Can you work these out from the model? Positions are in its coordinate system, mm. A direction names the side the tool comes from. Give positions to 0.01 mm unless a question says otherwise; leave off trailing zeros. Loops run counter-clockwise (first coordinate to the right, second up) from the corner with the lowest first, then second, coordinate; pieces in that order, holes last. Notation, with made-up numbers: (77, 57.5) - (131, 57.5) arc R23 cw to (131, 79.5) - close; hole circle Ø6 at (-9, 52). An arc over 180 degrees is marked (long way). Answer in a Markdown table with one row per item.
from build123d import *

# Parameters (mm, degrees)
SKETCH1_W            = 6.6
SKETCH1_H            = 11.95
BOSS_EXTRUDE1_DEPTH  = 5
SKETCH2_W            = 3.4
SKETCH2_H            = 0.5
CUT_EXTRUDE1_DEPTH   = 1.4
SKETCH3_W            = 2.2
SKETCH3_H            = 0.65
CUT_EXTRUDE2_DEPTH   = 7.1
SKETCH4_W            = 2.2
SKETCH4_H            = 0.25
BOSS_EXTRUDE2_DEPTH  = 0.5
SKETCH5_W            = 2.2
SKETCH5_H            = 0.25
BOSS_EXTRUDE3_DEPTH  = 0.6
SKETCH6_W            = 3.4
SKETCH6_H            = 0.5
CUT_EXTRUDE3_DEPTH   = 1.4
SKETCH7_W            = 2.2
SKETCH7_H            = 0.65
CUT_EXTRUDE4_DEPTH   = 7.1
SKETCH8_W            = 2.2
SKETCH8_H            = 0.25
BOSS_EXTRUDE4_DEPTH  = 0.5
SKETCH9_W            = 2.2
SKETCH9_H            = 0.25
BOSS_EXTRUDE5_DEPTH  = 0.6
CUT_EXTRUDE5_DEPTH   = 3.6
CUT_EXTRUDE6_REACH   = 2.9
SKETCH12_W           = 2.2
SKETCH12_H           = 2.6
CUT_EXTRUDE7_REACH   = 12.275
SKETCH13_W           = 1.85
SKETCH13_H           = 4.85
SKETCH14_W           = 2.5
SKETCH14_H           = 4.25
CUT_EXTRUDE8_DEPTH   = 1.65
CUT_EXTRUDE9_REACH   = 2.9
SKETCH16_W           = 2.2
SKETCH16_H           = 2.6
CUT_EXTRUDE10_REACH  = 12.275
SKETCH17_W           = 1.85
SKETCH17_H           = 4.85
SKETCH18_W           = 2.5
SKETCH18_H           = 4.25
CUT_EXTRUDE11_DEPTH  = 1.65
CUT_EXTRUDE12_REACH  = 6.85
SKETCH20_W           = 0.8
SKETCH20_H           = 3.6
SKETCH21_W           = 0.8
SKETCH21_H           = 1.9
CUT_EXTRUDE13_DEPTH  = 2.675
SKETCH22_W           = 0.8
SKETCH22_H           = 1.9
CUT_EXTRUDE14_DEPTH  = 2.675
SKETCH23_W           = 0.5
SKETCH23_H           = 0.5
BOSS_EXTRUDE6_DEPTH  = 2
SKETCH24_W           = 0.5
SKETCH24_H           = 0.5
BOSS_EXTRUDE7_DEPTH  = 2
SKETCH25_W           = 0.5
SKETCH25_H           = 0.5
BOSS_EXTRUDE8_DEPTH  = 2
SKETCH26_W           = 0.5
SKETCH26_H           = 0.5
BOSS_EXTRUDE9_DEPTH  = 2
SKETCH27_W           = 0.5
SKETCH27_H           = 0.5
BOSS_EXTRUDE10_DEPTH = 3.3
SKETCH28_W           = 0.5
SKETCH28_H           = 0.5
BOSS_EXTRUDE11_DEPTH = 3.3
SKETCH29_W           = 0.5
SKETCH29_H           = 0.5
BOSS_EXTRUDE12_DEPTH = 3.3
SKETCH30_W           = 0.5
SKETCH30_H           = 0.5
BOSS_EXTRUDE13_DEPTH = 3.3
DRAFT1_ANGLE         = 45


with BuildPart() as part:
    # Sketch1 → Boss-Extrude1 (new body)
    with BuildSketch(Plane(origin=(-5, 0, 0), x_dir=(0, -1, 0), z_dir=(-1, 0, 0))):
        with Locations((-3.3, 0)):
            Rectangle(SKETCH1_W, SKETCH1_H)
    extrude(amount=-BOSS_EXTRUDE1_DEPTH)

    # Sketch2 → Cut-Extrude1 (cut)
    with BuildSketch(Plane.XY.offset(5.975)):
        with Locations((-2.5, 0.25)):
            Rectangle(SKETCH2_W, SKETCH2_H)
    extrude(amount=-CUT_EXTRUDE1_DEPTH, mode=Mode.SUBTRACT)

    # Sketch3 → Cut-Extrude2 (cut, through all)
    with BuildSketch(Plane.XZ.offset(-0.5)):
        with Locations((-2.5, 5.65)):
            Rectangle(SKETCH3_W, SKETCH3_H)
    extrude(amount=-CUT_EXTRUDE2_DEPTH, mode=Mode.SUBTRACT)

    # Sketch4 → Boss-Extrude2 (add)
    with BuildSketch(Plane.XZ.offset(-0.5)):
        with Locations((-2.5, 5.2)):
            Rectangle(SKETCH4_W, SKETCH4_H)
    extrude(amount=BOSS_EXTRUDE2_DEPTH)

    # Sketch5 → Boss-Extrude3 (add)
    with BuildSketch(Plane.XY.offset(5.325)):
        with Locations((-2.5, 0.125)):
            Rectangle(SKETCH5_W, SKETCH5_H)
    extrude(amount=BOSS_EXTRUDE3_DEPTH)

    # Sketch6 → Cut-Extrude3 (cut)
    with BuildSketch(Plane(origin=(0, 0, -5.975), x_dir=(-1, 0, 0), z_dir=(0, 0, -1))):
        with Locations((2.5, 0.25)):
            Rectangle(SKETCH6_W, SKETCH6_H)
    extrude(amount=-CUT_EXTRUDE3_DEPTH, mode=Mode.SUBTRACT)

    # Sketch7 → Cut-Extrude4 (cut, through all)
    with BuildSketch(Plane.XZ.offset(-0.5)):
        with Locations((-2.5, -5.65)):
            Rectangle(SKETCH7_W, SKETCH7_H)
    extrude(amount=-CUT_EXTRUDE4_DEPTH, mode=Mode.SUBTRACT)

    # Sketch8 → Boss-Extrude4 (add)
    with BuildSketch(Plane.XZ.offset(-0.5)):
        with Locations((-2.5, -5.2)):
            Rectangle(SKETCH8_W, SKETCH8_H)
    extrude(amount=BOSS_EXTRUDE4_DEPTH)

    # Sketch9 → Boss-Extrude5 (add)
    with BuildSketch(Plane(origin=(0, 0, -5.325), x_dir=(-1, 0, 0), z_dir=(0, 0, -1))):
        with Locations((2.5, 0.125)):
            Rectangle(SKETCH9_W, SKETCH9_H)
    extrude(amount=BOSS_EXTRUDE5_DEPTH)

    # Sketch10 → Cut-Extrude5 (cut)
    with BuildSketch(Plane(origin=(0, 0, -1.8), x_dir=(-1, 0, 0), z_dir=(0, 0, -1))):
        Polygon((5, 2.35), (5, 6.6), (0.7, 6.6), (0.7, 1.75), (2.55, 1.75), (2.55, 2.35), align=None)
    extrude(amount=-CUT_EXTRUDE5_DEPTH, mode=Mode.SUBTRACT)

    # Sketch12 → Cut-Extrude6 (cut, up to next)
    with BuildSketch(Plane(origin=(0, 0, 5.075), x_dir=(-1, 0, 0), z_dir=(0, 0, -1)), mode=Mode.PRIVATE) as cut_extrude6_sk1:
        with Locations((2.5, 5.3)):
            Rectangle(SKETCH12_W, SKETCH12_H)
    cut_extrude6_tool1 = extrude(cut_extrude6_sk1.sketch, amount=-CUT_EXTRUDE6_REACH, mode=Mode.PRIVATE) & part.part
    add(cut_extrude6_tool1.solids().sort_by_distance((-2.5, 5.3, 5.075))[0], mode=Mode.SUBTRACT)

    # Sketch13 → Cut-Extrude7 (cut, up to next)
    with BuildSketch(Plane.XY.offset(4.3), mode=Mode.PRIVATE) as cut_extrude7_sk1:
        with Locations((-1.625, 4.175)):
            Rectangle(SKETCH13_W, SKETCH13_H)
    cut_extrude7_tool1 = extrude(cut_extrude7_sk1.sketch, amount=-CUT_EXTRUDE7_REACH, mode=Mode.PRIVATE) & part.part
    add(cut_extrude7_tool1.solids().sort_by_distance((-1.625, 4.175, 4.3))[0], mode=Mode.SUBTRACT)

    # Sketch14 → Cut-Extrude8 (cut)
    with BuildSketch(Plane(origin=(-2.55, 0, 0), x_dir=(0, 0, -1), z_dir=(1, 0, 0))):
        with Locations((-3.05, 4.475)):
            Rectangle(SKETCH14_W, SKETCH14_H)
    extrude(amount=-CUT_EXTRUDE8_DEPTH, mode=Mode.SUBTRACT)

    # Sketch16 → Cut-Extrude9 (cut, up to next)
    with BuildSketch(Plane.XY.offset(-5.075), mode=Mode.PRIVATE) as cut_extrude9_sk1:
        with Locations((-2.5, 5.3)):
            Rectangle(SKETCH16_W, SKETCH16_H)
    cut_extrude9_tool1 = extrude(cut_extrude9_sk1.sketch, amount=-CUT_EXTRUDE9_REACH, mode=Mode.PRIVATE) & part.part
    add(cut_extrude9_tool1.solids().sort_by_distance((-2.5, 5.3, -5.075))[0], mode=Mode.SUBTRACT)

    # Sketch17 → Cut-Extrude10 (cut, up to next)
    with BuildSketch(Plane(origin=(0, 0, -4.3), x_dir=(-1, 0, 0), z_dir=(0, 0, -1)), mode=Mode.PRIVATE) as cut_extrude10_sk1:
        with Locations((1.625, 4.175)):
            Rectangle(SKETCH17_W, SKETCH17_H)
    cut_extrude10_tool1 = extrude(cut_extrude10_sk1.sketch, amount=-CUT_EXTRUDE10_REACH, mode=Mode.PRIVATE) & part.part
    add(cut_extrude10_tool1.solids().sort_by_distance((-1.625, 4.175, -4.3))[0], mode=Mode.SUBTRACT)

    # Sketch18 → Cut-Extrude11 (cut)
    with BuildSketch(Plane(origin=(-2.55, 0, 0), x_dir=(0, 0, -1), z_dir=(1, 0, 0))):
        with Locations((3.05, 4.475)):
            Rectangle(SKETCH18_W, SKETCH18_H)
    extrude(amount=-CUT_EXTRUDE11_DEPTH, mode=Mode.SUBTRACT)

    # Sketch20 → Cut-Extrude12 (cut, up to next)
    with BuildSketch(Plane.XZ.offset(-1.75), mode=Mode.PRIVATE) as cut_extrude12_sk1:
        with Locations((-4.6, 0)):
            Rectangle(SKETCH20_W, SKETCH20_H)
    cut_extrude12_tool1 = extrude(cut_extrude12_sk1.sketch, amount=-CUT_EXTRUDE12_REACH, mode=Mode.PRIVATE) & part.part
    add(cut_extrude12_tool1.solids().sort_by_distance((-4.6, 1.75, 0))[0], mode=Mode.SUBTRACT)

    # Sketch21 → Cut-Extrude13 (cut, through all)
    with BuildSketch(Plane(origin=(0, 0, 4.3), x_dir=(-1, 0, 0), z_dir=(0, 0, -1))):
        with Locations((2.95, 5.65)):
            Rectangle(SKETCH21_W, SKETCH21_H)
    extrude(amount=-CUT_EXTRUDE13_DEPTH, mode=Mode.SUBTRACT)

    # Sketch22 → Cut-Extrude14 (cut, through all)
    with BuildSketch(Plane.XY.offset(-4.3)):
        with Locations((-2.95, 5.65)):
            Rectangle(SKETCH22_W, SKETCH22_H)
    extrude(amount=-CUT_EXTRUDE14_DEPTH, mode=Mode.SUBTRACT)

    # Sketch23 → Boss-Extrude6 (add)
    with BuildSketch(Plane(origin=(0, 0, 0), x_dir=(0, 0, -1), z_dir=(1, 0, 0))):
        with Locations((-3, 0.25)):
            Rectangle(SKETCH23_W, SKETCH23_H)
    extrude(amount=BOSS_EXTRUDE6_DEPTH)

    # Sketch24 → Boss-Extrude7 (add)
    with BuildSketch(Plane(origin=(0, 0, 0), x_dir=(0, 0, -1), z_dir=(1, 0, 0))):
        with Locations((-1, 0.25)):
            Rectangle(SKETCH24_W, SKETCH24_H)
    extrude(amount=BOSS_EXTRUDE7_DEPTH)

    # Sketch25 → Boss-Extrude8 (add)
    with BuildSketch(Plane(origin=(0, 0, 0), x_dir=(0, 0, -1), z_dir=(1, 0, 0))):
        with Locations((1, 0.25)):
            Rectangle(SKETCH25_W, SKETCH25_H)
    extrude(amount=BOSS_EXTRUDE8_DEPTH)

    # Sketch26 → Boss-Extrude9 (add)
    with BuildSketch(Plane(origin=(0, 0, 0), x_dir=(0, 0, -1), z_dir=(1, 0, 0))):
        with Locations((3, 0.25)):
            Rectangle(SKETCH26_W, SKETCH26_H)
    extrude(amount=BOSS_EXTRUDE9_DEPTH)

    # Sketch27 → Boss-Extrude10 (add)
    with BuildSketch(Plane(origin=(0, 2.35, 0), x_dir=(-1, 0, 0), z_dir=(0, 1, 0))):
        with Locations((3.1, -3)):
            Rectangle(SKETCH27_W, SKETCH27_H)
    extrude(amount=BOSS_EXTRUDE10_DEPTH)

    # Sketch28 → Boss-Extrude11 (add)
    with BuildSketch(Plane(origin=(0, 2.35, 0), x_dir=(-1, 0, 0), z_dir=(0, 1, 0))):
        with Locations((3.1, -1)):
            Rectangle(SKETCH28_W, SKETCH28_H)
    extrude(amount=BOSS_EXTRUDE11_DEPTH)

    # Sketch29 → Boss-Extrude12 (add)
    with BuildSketch(Plane(origin=(0, 2.35, 0), x_dir=(-1, 0, 0), z_dir=(0, 1, 0))):
        with Locations((3.1, 1)):
            Rectangle(SKETCH29_W, SKETCH29_H)
    extrude(amount=BOSS_EXTRUDE12_DEPTH)

    # Sketch30 → Boss-Extrude13 (add)
    with BuildSketch(Plane(origin=(0, 2.35, 0), x_dir=(-1, 0, 0), z_dir=(0, 1, 0))):
        with Locations((3.1, 3)):
            Rectangle(SKETCH30_W, SKETCH30_H)
    extrude(amount=BOSS_EXTRUDE13_DEPTH)

    # Draft1
    draft1_faces = [part.faces().sort_by_distance(p)[0] for p in [
        (-2.55, 2.05, 0),
    ]]
    draft(draft1_faces, Plane(origin=(-2.55, 2.35, 1.8), x_dir=(0, 0, 1), z_dir=(0, 1, 0)), DRAFT1_ANGLE)


solid = part.part
Q1. If I drill on line 1 (X direction, y = 5, z = -3); line 2 (X direction, y = 2.5, z = -2.25); line 3 (Z direction, x = -4.25, y = 2) (3 decimals), over which ranges is the centre line in solid material (lowest first)? Write a range as [from, to].
Checked values:
| item | result |
|---|---|
| line 1 | x = [-5, -4.2], [-3.35, -2.85], [-0.7, 0] |
| line 2 | x = [-5, -4.2], [-0.7, 0] |
| line 3 | z = [-5.975, -1.8], [1.8, 5.975] |
Q2. Imagine slicing it at D-D, the plane z = -0.25. Write out the boundary of the cut face in (x, y), and give its area (3 significant figures).
Checked values:
| item | result |
|---|---|
| outline | (-5, 0) - (0, 0) - (0, 6.6) - (-0.7, 6.6) - (-0.7, 1.75) - (-1.95, 1.75) - (-2.55, 2.35) - (-4.2, 2.35) - (-4.2, 1.75) - (-5, 1.75) - close |
| area | 13.3 mm² |
Q3. Imagine slicing it at B-B, the plane y = 6. Write out the boundary of the cut face in (x, z) (3 decimals).
Checked values:
| item | result |
|---|---|
| outline | (-5, -5.975) - (-3.6, -5.975) - (-3.6, -5.075) - (-3.35, -5.075) - (-3.35, -4.3) - (-4.2, -4.3) - (-4.2, -1.8) - (-5, -1.8) - close; (-5, 1.8) - (-4.2, 1.8) - (-4.2, 4.3) - (-3.35, 4.3) - (-3.35, 5.075) - (-3.6, 5.075) - (-3.6, 5.975) - (-5, 5.975) - close; (-2.55, -5.075) - (-1.4, -5.075) - (-1.4, -5.975) - (0, -5.975) - (0, 5.975) - (-1.4, 5.975) - (-1.4, 5.075) - (-2.55, 5.075) - (-2.55, 4.3) - (-0.7, 4.3) - (-0.7, -4.3) - (-2.55, -4.3) - close |
Q4. On a 3-axis mill with a long thin cutter (end or side, diameter ignored), from which of +Z, -Z, +X, -X, +Y, -Y can I reach the whole of each face in a straight line? I mean faces 1 (the face through (-0.7, 4, 0)), 2 (the face through (-1.4, 3.5, -5.5)), 3 (the face through (-4.6, 1.75, 0)). Say none if no direction works.
Checked values:
| item | result |
|---|---|
| face 1 | +Y |
| face 2 | -Z, +Y |
| face 3 | -X, +Y |
Q5. Imagine slicing it at A-A, the plane x = 1.25. Write out the boundary of the cut face in (y, z), and give its area (3 significant figures).
Checked values:
| item | result |
|---|---|
| outline | (0, -3.25) - (0.5, -3.25) - (0.5, -2.75) - (0, -2.75) - close; (0, -1.25) - (0.5, -1.25) - (0.5, -0.75) - (0, -0.75) - close; (0, 0.75) - (0.5, 0.75) - (0.5, 1.25) - (0, 1.25) - close; (0, 2.75) - (0.5, 2.75) - (0.5, 3.25) - (0, 3.25) - close |
| area | 1.00 mm² |
Q6. Imagine slicing it at C-C, the plane y = 1.5. Write out the boundary of the cut face in (x, z) (3 decimals).
Checked values:
| item | result |
|---|---|
| outline | (-5, -5.975) - (-3.6, -5.975) - (-3.6, -5.325) - (-1.4, -5.325) - (-1.4, -5.975) - (0, -5.975) - (0, 5.975) - (-1.4, 5.975) - (-1.4, 5.325) - (-3.6, 5.325) - (-3.6, 5.975) - (-5, 5.975) - close |
Q7. If we mould it in two halves opening along Z, with no side actions, what happens to faces 4 (the face through (-1, 3, -5.975)), 5 (the face through (-4.2, 5, 3)), 6 (the face through (-4.4, 6.6, -4.4))? For each: released by +Z, released by -Z, zero draft, split by the parting line, or undercut.
Checked values:
| item | result |
|---|---|
| face 4 | released by -Z |
| face 5 | undercut |
| face 6 | zero draft |
Q8. For pin 1 (0.8 mm diameter, centred on x = -3.5, z = -1, fed in from +Y); pin 2 (1.8 mm diameter, centred on x = -2.5, y = 6, fed in from +Z) (3 decimals); pin 3 (0.6 mm diameter, centred on x = -3, y = 4.5, fed in from -Z) (3 decimals), each with a flat end and sliding along its axis, tell me the tip position at first contact or that it passes through.
Checked values:
| item | result |
|---|---|
| pin 1 | stops at y = 5.65 |
| pin 2 | stops at z = 5.075 |
| pin 3 | stops at z = -5.075 |
